Autodesk Inventor part; units mm, degrees
ref_plane "YZ Plane" through (0, 0, 0) normal (1, 0, 0) x (0, 1, 0)
ref_plane "XZ Plane" through (0, 0, 0) normal (0, 1, 0) x (-1, 0, 0)
ref_plane "XY Plane" through (0, 0, 0) normal (0, 0, 1) x (1, 0, 0)
sketch "スケッチ1" plane through (0, 0, 0) normal (0, 0, 1) x (1, 0, 0)
  circle A0 centre (0, 0) radius 1.5
  circle A1 centre (0, 0) radius 2.5
  dimension "d0" = 3
  dimension "d1" = 5
extrude "押し出し1" add sketch "スケッチ1" along normal blind 3
chamfer "面取り1" distance 0.5 angle 45 1 edges at (-2.5, 0, 3)
sketch "スケッチ2" plane through (0, 0, 0) normal (0, 0, -1) x (-1, 0, 0)
  circle A0 centre (0, 0) radius 1.5
  circle A1 centre (0, 0) radius 4
  dimension "d7" = 8
extrude "押し出し2" add sketch "スケッチ2" along normal blind 1
properties part number "オイレスw3f3-5a" material "アセタール樹脂、黒"
Design review of the part built by this model. Coordinates are the model's own, in mm. A direction names the side the tool comes from. Round coordinates to 2 decimals unless told otherwise and drop trailing zeros. Write each loop counter-clockwise with the first axis right and the second up, starting at its lowest first coordinate (ties: lowest second). Pieces come first, ordered by that corner, then holes. Notation, with made-up numbers: M 86,44.25 L 121,44.25 A25 ccw 121,77.25 Z; hole C 24,-17.5 d1. An arc over 180 degrees is marked long. One line per item, written item: value. Start each with the question number.
1. To check wall thickness, follow probe 1 along Y at (x, z) = (0, -0.3); probe 2 along Y at (x, z) = (0, 2.2); probe 3 along Z at (x, y) = (-2.25, -2.75). State the ranges of each line that lie inside material, in increasing order. Write a range as from..to.
2. Clearance check with a flat-ended pin moving along its axis: P1, Ø4, axis at x = 3, y = 0.5, coming from the +Z side. State where the tip first meets the part, or that it passes through.
3. Take a section at C-C on z = 0.6. State the section outline as (x, y) points.
4. For faces 1 (the face through (0.867, 3.905, -0.493)), 2 (the face through (-0.54, 2.44, 1.23)), list the 3-axis set-ups (+Z, -Z, +X, -X, +Y, -Y) from which the entire face can be reached by the end or side of a thin tool; tool diameter is ignored.
5. Take a section at D-D on z = 2.6. State the section outline as (x, y) points.
6. Take a section at A-A on x = 0. State the section outline as (y, z) points.
Computed:
1. probe 1: y = -4..-1.5, 1.5..4
1. probe 2: y = -2.5..-1.5, 1.5..2.5
1. probe 3: z = -1..0
2. P1: stops at z = 3
3. outline: C 0,0 d5; hole C 0,0 d3
4. face 1: +Z, -Z
4. face 2: +Z
5. outline: C 0,0 d4.8; hole C 0,0 d3
6. outline: M -4,-1 L -1.5,-1 L -1.5,3 L -2,3 L -2.5,2.5 L -2.5,0 L -4,0 Z; M 1.5,-1 L 4,-1 L 4,0 L 2.5,0 L 2.5,2.5 L 2,3 L 1.5,3 Z
